```python
from build123d import *

# Parameters (mm, degrees)
F0_W      = 534.8856896162
F0_H      = 573.5703483224
F1_DEPTH  = 6.35
F2_W      = 534.8856896162
F2_H      = 8.2960128784
F3_DEPTH  = 254
F4_W      = 534.8856896162
F4_H      = 11.1295878887
F5_DEPTH  = 254
F6_W      = 534.8856896162
F6_H      = 11.2980566919
F7_DEPTH  = 254
F8_W      = 10.6345191598
F8_H      = 555.1736503839
F8_H_2    = 277.0723737776
F9_DEPTH  = 254
F10_W     = 573.5703483224
F10_H     = 260.35
F11_DEPTH = 25.4
F12_W     = 12.9221528769
F12_H     = 254
F13_DEPTH = 558.8
F14_W     = 573.5703483224
F14_H     = 260.35
F15_DEPTH = 10.16
F16_W     = 15.8027634025
F16_H     = 260.35
F17_DEPTH = 690.88
F18_W     = 18.2235240936
F18_H     = 260.35
F19_DEPTH = 690.88
F20_W     = 12.0796486735
F20_H     = 260.35
F21_DEPTH = 690.88
F22_W     = 10.1929306984
F22_H     = 260.35
F23_DEPTH = 553.72
F24_W     = 11.8005871773
F24_H     = 260.35
F25_DEPTH = 551.18
F26_W     = 571.6413035989
F26_H     = 260.35
F27_DEPTH = 43.18
F28_W     = 547.8762835264
F28_H     = 13.0373798311
F29_DEPTH = 688.34


with BuildPart() as f1:
    # F0 (on Top) → F1 (new body)
    with BuildSketch(Plane.XY):
        with Locations((-66.9661834836, 184.2964999378)):
            Rectangle(F0_W, F0_H)
    extrude(amount=F1_DEPTH)

    # F2 (on face) → F3 (join)
    with BuildSketch(Plane.XY.offset(6.35)):
        with Locations((-66.9661834836, -98.3406677842)):
            Rectangle(F2_W, F2_H)
    extrude(amount=F3_DEPTH)

    # F4 (on face) → F5 (join)
    with BuildSketch(Plane.XY.offset(6.35)):
        with Locations((-66.9661834836, 465.5168801546)):
            Rectangle(F4_W, F4_H)
    extrude(amount=F5_DEPTH)

    # F6 (on face) → F7 (join)
    with BuildSketch(Plane.XY.offset(6.35)):
        with Locations((-66.9661834836, 177.2306840867)):
            Rectangle(F6_W, F6_H)
    extrude(amount=F7_DEPTH)

    # F8 (on face) → F9 (join)
    with BuildSketch(Plane.XY.offset(6.35)):
        with Locations((-72.2834430635, 182.3652610183)):
            Rectangle(F8_W, F8_H)
        with Locations((-72.2834430635, 321.4158993214)):
            Rectangle(F8_W, F8_H_2)
    extrude(amount=F9_DEPTH)

    # F10 (on face) → F11 (join)
    with BuildSketch(Plane.YZ.offset(200.4766613245)):
        with Locations((184.2964999378, 130.175)):
            Rectangle(F10_W, F10_H)
    extrude(amount=F11_DEPTH)

    # F12 (on face) → F13 (join)
    with BuildSketch(Plane.XZ.offset(-459.9520862103)):
        with Locations((-162.5997051597, 133.35)):
            Rectangle(F12_W, F12_H)
    extrude(amount=F13_DEPTH)

    # F14 (on face) → F15 (join)
    with BuildSketch(Plane(origin=(-334.4090282917, 0, 0), x_dir=(0, -1, 0), z_dir=(-1, 0, 0))):
        with Locations((-184.2964999378, 130.175)):
            Rectangle(F14_W, F14_H)
    extrude(amount=F15_DEPTH)

    # F16 (on face) → F17 (join)
    with BuildSketch(Plane(origin=(-344.5690282917, 0, 0), x_dir=(0, -1, 0), z_dir=(-1, 0, 0))):
        with Locations((94.5872925222, 130.175)):
            Rectangle(F16_W, F16_H)
    extrude(amount=F17_DEPTH)

    # F18 (on face) → F19 (join)
    with BuildSketch(Plane(origin=(-344.5690282917, 0, 0), x_dir=(0, -1, 0), z_dir=(-1, 0, 0))):
        with Locations((-461.9699120522, 130.175)):
            Rectangle(F18_W, F18_H)
    extrude(amount=F19_DEPTH)

    # F20 (on face) → F21 (join)
    with BuildSketch(Plane(origin=(-344.5690282917, 0, 0), x_dir=(0, -1, 0), z_dir=(-1, 0, 0))):
        with Locations((-177.0462952554, 130.175)):
            Rectangle(F20_W, F20_H)
    extrude(amount=F21_DEPTH)

    # F22 (on face) → F23 (join)
    with BuildSketch(Plane.XZ.offset(-452.8581500053)):
        with Locations((-549.6869385242, 130.175)):
            Rectangle(F22_W, F22_H)
    extrude(amount=F23_DEPTH)

    # F24 (on face) → F25 (join)
    with BuildSketch(Plane(origin=(0, -86.685910821, 0), x_dir=(-1, 0, 0), z_dir=(0, 1, 0))):
        with Locations((767.846673727, 130.175)):
            Rectangle(F24_W, F24_H)
    extrude(amount=F25_DEPTH)

    # F26 (on face) → F27 (join)
    with BuildSketch(Plane(origin=(-1035.4490282917, 0, 0), x_dir=(0, -1, 0), z_dir=(-1, 0, 0))):
        with Locations((-183.331977576, 130.175)):
            Rectangle(F26_W, F26_H)
    extrude(amount=-F27_DEPTH)

    # F28 (on face) → F29 (join)
    with BuildSketch(Plane(origin=(-344.5690282917, 0, 0), x_dir=(0, -1, 0), z_dir=(-1, 0, 0))):
        with Locations((-187.2522309422, 6.5186899155)):
            Rectangle(F28_W, F28_H)
    extrude(amount=F29_DEPTH)


solid = f1.part
```
Part model, mm, in its own coordinate system. Round coordinates to 2 decimals unless told otherwise and drop trailing zeros. Loops run counter-clockwise (first coordinate to the right, second up) from the corner with the lowest first, then second, coordinate; pieces in that order, holes last.
Item 1: Drop flat-ended pins along their axis: P1, Ø3, axis at x = -171.5, y = 218.5, coming from the +Z side; P2, Ø4, axis at x = -618, y = 207.5, coming from the +Z side. Give the stop position or say it passes through.
Item 2: Drill centre lines: line 1 (Y direction, x = 2, z = 237); line 2 (Y direction, x = -652, z = 62); line 3 (Z direction, x = -187, y = -37.5). Where is each one in solid material? Low to high.
Item 3: Cut at D-D, the plane x = -120.5. Give the cut face in (y, z), then the cut area to 3 significant figures.
Item 4: Mould opens along X. For faces 1 (the face through (225.877, 180, 132)), 2 (the face through (-168, 162, 260.35)), 3 (the face through (-117, 182.88, 132)) say: +X half, -X half, draft (parallel to the pull), parting line (faces both ways), or undercut.
Item 5: Cut at A-A, the plane x = -915.5. Give the cut face in (y, z), then the cut area to 3 significant figures.
Item 6: Cut at B-B, the plane y = 217.5. Give the cut face in (x, z).
Item 7: Cut at C-C, the plane z = 63. State how many separate pieces and enclosed holes the cut face has, then the cut area to 3 significant figures.
A:
1. P1: stops at z = 6.35
1. P2: stops at z = 13.04
2. line 1: y = -102.49 to -94.19, 171.58 to 182.88, 459.95 to 471.08
2. line 2: y = -102.49 to -86.69, 171.01 to 183.09, 452.86 to 471.08
2. line 3: z = 0 to 6.35
3. outline: (-102.49, 0) - (471.08, 0) - (471.08, 260.35) - (459.95, 260.35) - (459.95, 6.35) - (182.88, 6.35) - (182.88, 260.35) - (171.58, 260.35) - (171.58, 6.35) - (-94.19, 6.35) - (-94.19, 260.35) - (-102.49, 260.35) - close
3. area: 11,400 mm2
4. face 1: +X half
4. face 2: draft
4. face 3: undercut
5. outline: (-102.49, 0) - (471.08, 0) - (471.08, 260.35) - (452.86, 260.35) - (452.86, 13.04) - (183.09, 13.04) - (183.09, 260.35) - (171.01, 260.35) - (171.01, 13.04) - (-86.69, 13.04) - (-86.69, 260.35) - (-102.49, 260.35) - close
5. area: 18,900 mm2
6. outline: (-1035.45, 0) - (225.88, 0) - (225.88, 260.35) - (200.48, 260.35) - (200.48, 6.35) - (-66.97, 6.35) - (-66.97, 260.35) - (-77.6, 260.35) - (-77.6, 6.35) - (-156.14, 6.35) - (-156.14, 260.35) - (-169.06, 260.35) - (-169.06, 6.35) - (-334.41, 6.35) - (-334.41, 260.35) - (-344.57, 260.35) - (-344.57, 13.04) - (-544.59, 13.04) - (-544.59, 260.35) - (-554.78, 260.35) - (-554.78, 13.04) - (-761.95, 13.04) - (-761.95, 260.35) - (-773.75, 260.35) - (-773.75, 13.04) - (-992.27, 13.04) - (-992.27, 260.35) - (-1035.45, 260.35) - close
7. separate pieces: 1
7. enclosed holes: 12
7. area: 116,000 mm2
